Autodesk Inventor part; units mm, degrees
ref_plane "YZ Plane" through (0, 0, 0) normal (1, 0, 0) x (0, 1, 0)
ref_plane "XZ Plane" through (0, 0, 0) normal (0, 1, 0) x (-1, 0, 0)
ref_plane "XY Plane" through (0, 0, 0) normal (0, 0, 1) x (1, 0, 0)
sketch "Esquisse1" plane through (0, 0, 0) normal (0, 0, 1) x (1, 0, 0)
  circle A0 centre (0, 0) radius 63
  circle A1 centre (0, 0) radius 60
  circle A2 centre (0, 0) radius 54
  line L0 (-25.9421, 2.5) -> (-53.9421, 2.5)
  line L1 (-25.9421, -2.5) -> (-53.9421, -2.5)
  line L2 (-20.9421, 0) -> (-20.9421, 14.5)
  line L3 (-25.9421, 14.5) -> (-25.9421, 2.5)
  line L4 (-20.9421, 0) -> (-20.9421, -14.5)
  line L5 (-25.9421, -14.5) -> (-25.9421, 2.5)
  arc A3 (-25.9421, -14.5) -> (-20.9421, -14.5) centre (-23.4421, -14.5) ccw
  arc A4 (-20.9421, 14.5) -> (-25.9421, 14.5) centre (-23.4421, 14.5) ccw
  line L6 (0, 0) -> (0, 11.8583)
  line L7 (25.9421, 2.5) -> (53.9421, 2.5)
  line L8 (25.9421, -2.5) -> (53.9421, -2.5)
  line L9 (20.9421, 0) -> (20.9421, 14.5)
  line L10 (25.9421, 14.5) -> (25.9421, 2.5)
  line L11 (20.9421, 0) -> (20.9421, -14.5)
  line L12 (25.9421, -14.5) -> (25.9421, 14.5)
  arc A5 (20.9421, -14.5) -> (25.9421, -14.5) centre (23.4421, -14.5) ccw
  arc A6 (25.9421, 14.5) -> (20.9421, 14.5) centre (23.4421, 14.5) ccw
  line L13 (25.9421, 2.5) -> (56.5559, 2.5)
  line L14 (56.5559, 2.5) -> (56.5559, -2.5)
  line L15 (56.5559, -2.5) -> (25.9421, -2.5)
  line L16 (25.9421, -2.5) -> (25.9421, 2.5)
  dimension "d0" = 126
  dimension "d1" = 120
  dimension "d2" = 108
  dimension "d3" = 28
  dimension "d6" = 14.5
  dimension "d8" = 5
extrude "Extrusion1" add sketch "Esquisse1" along normal blind 5 contours A0
extrude "Extrusion2" add sketch "Esquisse1" along normal blind 1.7 contours A1 | A2 L8 L12 L7 | A2 L13 L14 L15 | L0 L5 L1 A2
sketch "Esquisse3" plane through (0, 0, 0) normal (0, 0, -1) x (-1, 0, 0)
  line L0 (20.9421, 0) -> (20.9421, 14.5)
  line L1 (20.9421, 0) -> (20.9421, -14.5)
  arc A0 (20.9421, -14.5) -> (25.9421, -14.5) centre (23.4421, -14.5) ccw
  line L2 (25.9421, -14.5) -> (25.9421, 2.5)
  line L3 (25.9421, 14.5) -> (25.9421, 2.5)
  arc A1 (25.9421, 14.5) -> (20.9421, 14.5) centre (23.4421, 14.5) ccw
  arc A2 (-20.9421, 14.5) -> (-25.9421, 14.5) centre (-23.4421, 14.5) ccw
  line L4 (-25.9421, 14.5) -> (-25.9421, 2.5)
  line L5 (-25.9421, -14.5) -> (-25.9421, 14.5)
  arc A3 (-25.9421, -14.5) -> (-20.9421, -14.5) centre (-23.4421, -14.5) ccw
  line L6 (-20.9421, 0) -> (-20.9421, -14.5)
  line L7 (-20.9421, 0) -> (-20.9421, 14.5)
  point P0 (0, 0)
extrude "Extrusion3" add sketch "Esquisse3" against normal blind 3
fillet "Congé1" radius 1 3 edges at (25.9421, 0, 1.7) (25.9421, -2.5, 0.85) (25.9421, 2.5, 0.85)
fillet "Congé2" radius 1 3 edges at (-25.9421, 0, 1.7) (-25.9421, -2.5, 0.85) (-25.9421, 2.5, 0.85)
fillet "Congé3" radius 1 4 edges at (53.9421, 2.5, 0.85) (53.9421, -2.5, 0.85) (-53.9421, 2.5, 0.85) (-53.9421, -2.5, 0.85)
sketch "Esquisse4" plane through (0, 0, 0) normal (0, 0, -1) x (-1, 0, 0)
  arc A0 (53.8821, 3.566) -> (-53.8821, 3.566) centre (0, 0) ccw
  arc A1 (-53.8821, -3.566) -> (53.8821, -3.566) centre (0, 0) ccw
  arc A2 (53.8821, 3.566) -> (-53.8821, 3.566) centre (0, 0) ccw
  arc A3 (52.8843, 2.5) -> (53.8821, 3.566) centre (52.8843, 3.5) ccw
  line L0 (52.8843, 2.5) -> (26.9421, 2.5)
  arc A4 (25.9421, 3.5) -> (26.9421, 2.5) centre (26.9421, 3.5) ccw
  line L1 (25.9421, 3.5) -> (25.9421, 14.5)
  arc A5 (25.9421, 14.5) -> (20.9421, 14.5) centre (23.4421, 14.5) ccw
  line L2 (20.9421, 14.5) -> (20.9421, -14.5)
  arc A6 (20.9421, -14.5) -> (25.9421, -14.5) centre (23.4421, -14.5) ccw
  line L3 (25.9421, -14.5) -> (25.9421, -3.5)
  arc A7 (26.9421, -2.5) -> (25.9421, -3.5) centre (26.9421, -3.5) ccw
  line L4 (26.9421, -2.5) -> (52.8843, -2.5)
  arc A8 (53.8821, -3.566) -> (52.8843, -2.5) centre (52.8843, -3.5) ccw
  arc A9 (-53.8821, -3.566) -> (53.8821, -3.566) centre (0, 0) ccw
  arc A10 (-52.8843, -2.5) -> (-53.8821, -3.566) centre (-52.8843, -3.5) ccw
  line L5 (-26.9421, -2.5) -> (-52.8843, -2.5)
  arc A11 (-25.9421, -3.5) -> (-26.9421, -2.5) centre (-26.9421, -3.5) ccw
  line L6 (-25.9421, -3.5) -> (-25.9421, -14.5)
  arc A12 (-25.9421, -14.5) -> (-20.9421, -14.5) centre (-23.4421, -14.5) ccw
  line L7 (-20.9421, -14.5) -> (-20.9421, 14.5)
  arc A13 (-20.9421, 14.5) -> (-25.9421, 14.5) centre (-23.4421, 14.5) ccw
  line L8 (-25.9421, 14.5) -> (-25.9421, 3.5)
  arc A14 (-26.9421, 2.5) -> (-25.9421, 3.5) centre (-26.9421, 3.5) ccw
  line L9 (-52.8843, 2.5) -> (-26.9421, 2.5)
  arc A15 (-53.8821, 3.566) -> (-52.8843, 2.5) centre (-52.8843, 3.5) ccw
  circle A16 centre (0, 0) radius 63
  line L10 (32.9786, 41.9728) -> (-33, 41.9728)
  line L11 (-33, 41.9728) -> (-33, -42)
  line L12 (-33, -42) -> (32.9786, -42)
  line L13 (32.9786, -42) -> (32.9786, 41.9728)
  line L14 (32.9786, 32.8) -> (-33, 32.8)
  line L15 (32.9786, -32.8) -> (-33, -32.8)
  line L16 (-33.3624, -42.4612) -> (38.9228, 49.5381)
  line L17 (33.3492, -42.4716) -> (-38.936, 49.5277)
  line L18 (-33.2831, 42.3332) -> (-36.4284, 39.8619)
  line L19 (-33.2831, 42.3332) -> (-30.1379, 44.8045)
  arc A17 (-30.1379, 44.8045) -> (-36.4284, 39.8619) centre (-32.5624, 41.4158) ccw
  line L20 (33.2707, 42.3445) -> (30.1254, 44.8158)
  line L21 (33.2707, 42.3445) -> (36.416, 39.8733)
  line L22 (33.2831, -42.3332) -> (36.4284, -39.8619)
  line L23 (33.2831, -42.3332) -> (30.1379, -44.8045)
  arc A18 (30.1379, -44.8045) -> (36.4284, -39.8619) centre (32.5624, -41.4158) ccw
  arc A19 (36.416, 39.8733) -> (30.1254, 44.8158) centre (32.5499, 41.4272) ccw
  line L24 (-33.2707, -42.3445) -> (-36.416, -39.8733)
  arc A20 (-36.416, -39.8733) -> (-30.1254, -44.8158) centre (-32.5499, -41.4272) ccw
  line L25 (-33.2707, -42.3445) -> (-30.1254, -44.8158)
  arc A21 (-53.8821, -3.566) -> (53.8821, -3.566) centre (0, 0) ccw
  line L26 (-38.5851, -37.7782) -> (-27.5766, -46.4277)
  arc A22 (-38.5851, -37.7782) -> (-27.5766, -46.4277) centre (-31.4173, -39.9857) ccw
  line L27 (-38.5969, 37.7661) -> (-27.5885, 46.4156)
  arc A23 (-27.5885, 46.4156) -> (-38.5969, 37.7661) centre (-31.4292, 39.9736) ccw
  line L28 (27.5621, -46.4363) -> (38.5705, -37.7868)
  arc A24 (27.5621, -46.4363) -> (38.5705, -37.7868) centre (31.4028, -39.9943) ccw
  line L29 (27.5766, 46.4277) -> (38.5851, 37.7782)
  arc A25 (38.5851, 37.7782) -> (27.5766, 46.4277) centre (31.4173, 39.9857) ccw
  point P0 (-35.1366, 44.6921)
  point P1 (35.1242, 44.7035)
  point P2 (33, -41.9728)
  point P3 (35.1366, -44.6921)
  point P4 (-32.9786, -41.9728)
  point P5 (-35.1242, -44.7035)
  point P6 (-38.9228, -49.5381)
  dimension "d42" = 33
  dimension "d43" = 42
  dimension "d44" = 4
  dimension "d45" = 4
  dimension "d46" = 3
  dimension "d47" = 65.9786
  dimension "d48" = 83.9728
  dimension "d53" = 4
  dimension "d54" = 4
  dimension "d55" = 3
  dimension "d58" = 360
  dimension "d62" = 360
  dimension "d80" = 7
  dimension "d81" = 14
  dimension "d82" = 7.5
  dimension "d83" = 14
  dimension "d84" = 7
  dimension "d85" = 7.5
  dimension "d86" = 14
  dimension "d87" = 7
  dimension "d88" = 7.5
  dimension "d89" = 14
  dimension "d90" = 7
  dimension "d91" = 7.5
extrude "Extrusion4" cut sketch "Esquisse4" against normal blind 10 contours L25 A1 L16 | L16 A1 L24 | A20 A1
extrude "Extrusion5" cut sketch "Esquisse4" against normal blind 10 contours L18 A0 L17 | A0 A17 L17 picked at (-34.5217, 42.711)
extrude "Extrusion6" cut sketch "Esquisse4" against normal blind 10 contours L19 L17 A0 | A0 L17 A17 picked at (-33.3576, 43.626)
extrude "Extrusion7" cut sketch "Esquisse4" against normal blind 10 contours L21 L16 A0 | A0 L16 A19 picked at (34.5088, 42.7218)
extrude "Extrusion8" cut sketch "Esquisse4" against normal blind 10 contours A18 A1 | A1 L17 L23 L22 | L17 A1 L23
extrude "Extrusion9" cut sketch "Esquisse4" against normal blind 10 contours L16 L20 A0 | A0 A19 L16 picked at (33.3443, 43.6367)
fillet "Congé4" radius 4 6 edges at (36.416, -39.8733, 0.85) (30.1254, -44.8158, 0.85) (36.4284, 39.8619, 0.85) (-36.416, 39.8733, 0.85) (-30.14, -44.806, 0.85) (-36.4284, -39.8619, 0.85)
extrude "Extrusion10" cut sketch "Esquisse4" against normal blind 10 contours A24 A1 A18 | A1 L22 L23 L17 L28 A24 | L17 L23 A1 L28
extrude "Extrusion11" cut sketch "Esquisse4" against normal blind 10 contours L29 L16 L21 A0 | A0 A19 L16 A25 | L29 A0 L20 L16 | L16 A19 A0 A25
extrude "Extrusion12" cut sketch "Esquisse4" against normal blind 10 contours A23 L27 L17 L19 A0 | A0 A17 L17 A23 | L27 A0 L18 L17 | L17 A17 A0 A23
extrude "Extrusion13" cut sketch "Esquisse4" against normal blind 10 contours L26 A1 L25 L16 | L16 L24 A1 L26 | A22 A1 A20
fillet "Congé5" radius 4 8 edges at (38.5851, -37.7782, 0.85) (27.5766, -46.4277, 0.85) (-27.5621, -46.4363, 0.85) (-38.572, -37.7916, 0.85) (27.5927, 46.4181, 0.85) (38.5969, 37.7661, 0.85) (-38.5851, 37.7782, 0.85) (-27.5766, 46.4277, 0.85)
equation "\"d80\" = 0.5 * d81"
equation "\"d90\" = 0.5 * d89"
properties part number "bumper_modified2" material "Plastique ABS"
The model under review builds one solid part; all positions refer to its coordinate system, in mm. A direction names the side the tool comes from. Give positions to 0.01 mm unless a question says otherwise; leave off trailing zeros. Write each loop counter-clockwise with the first axis right and the second up, starting at its lowest first coordinate (ties: lowest second). Pieces come first, ordered by that corner, then holes. Notation, with made-up numbers: (8.25, 86) -> (40.25, 86) arc R8 cw to (40.25, 93) -> close; hole circle Ø3 at (76, 81.25). An arc over 180 degrees is marked (long way). Put each result on its own line as item: value.
(1) We need section A-A, the plane x = 0. Give the boundary of the cut face in (y, z), and give its area (3 significant figures).
Results are:
outline: (-63, 0) -> (-54, 0) -> (-54, 1.7) -> (-60, 1.7) -> (-60, 5) -> (-63, 5) -> close; (54, 0) -> (63, 0) -> (63, 5) -> (60, 5) -> (60, 1.7) -> (54, 1.7) -> close
area: 50.4 mm²
(2) The part is to be moulded in two halves that separate along Y. For faces 4 (the cylindrical face through (-49.785, 20.915, 0.838)), 5 (the flat face through (-23, 0, 0)), say which applies: pulls with the +Y half, pulls with the -Y half, needs draft (parallel to the pull), parting line crosses it, or undercut.
Results are:
face 4: undercut
face 5: needs draft
(3) For pin 1 Ø2.5 at (x, y) = (-24, -4) entering from +Z; pin 2 Ø1.5 at (y, z) = (-4, 2) entering from +X; pin 3 Ø0.5 at (x, z) = (-41, 1) entering from -Y, all flat-tipped, find the tip position at first contact; note any pin that passes through.
Results are:
pin 1: z = 3
pin 2: x = 62.92
pin 3: y = -48.05
(4) We need section B-B, the plane y = 0. Give the boundary of the cut face in (x, z).
Results are:
outline: (-63, 0) -> (-20.94, 0) -> (-20.94, 3) -> (-25.94, 3) -> (-25.94, 2.7) arc R1 cw to (-26.94, 1.7) -> (-60, 1.7) -> (-60, 5) -> (-63, 5) -> close; (20.94, 0) -> (63, 0) -> (63, 5) -> (60, 5) -> (60, 1.7) -> (26.94, 1.7) arc R1 cw to (25.94, 2.7) -> (25.94, 3) -> (20.94, 3) -> close
(5) We need section C-C, the plane x = -32. Give the boundary of the cut face in (y, z).
Results are:
outline: (-54.27, 0) -> (-47.47, 0) -> (-47.47, 1.7) -> (-50.75, 1.7) -> (-50.75, 5) -> (-54.27, 5) -> close; (-2.5, 0) -> (2.5, 0) -> (2.5, 1.7) -> (-2.5, 1.7) -> close; (47.46, 0) -> (54.27, 0) -> (54.27, 5) -> (50.75, 5) -> (50.75, 1.7) -> (47.46, 1.7) -> close
(6) Tool access review of faces 1 (the cylindrical face through (-59.94, -2.64, 3.33)), 2 (the flat face through (56, -23, 5)), 3 (the cylindrical face through (-23.4, -17, 1.5)): name each direction out of +Z, -Z, +X, -X, +Y, -Y from which nothing blocks a thin tool from reaching the whole face with its end or side.
Results are:
face 1: +Z
face 2: +Z, +X, -X, +Y, -Y
face 3: +Z, -Z
(7) To check wall thickness, follow probe 1 along Y at (x, z) = (-22, 1.05); probe 2 along Y at (x, z) = (0, 2.6); probe 3 along X at (y, z) = (-54, 4.55). State the ranges of each line that lie inside material, in increasing order. Write a range as from..to.
Results are:
probe 1: -59.03..-49.32, -16.54..16.54, 49.32..59.03
probe 2: -63..-60, 60..63
probe 3: -32.45..-26.15, 26.15..32.45
(8) We need section D-D, the plane y = -49.5. Give the boundary of the cut face in (x, z).
Results are:
outline: (-38.97, 0) -> (-21.58, 0) -> (-21.58, 1.7) -> (-33.91, 1.7) -> (-33.91, 5) -> (-38.97, 5) -> close; (21.58, 0) -> (38.97, 0) -> (38.97, 5) -> (33.91, 5) -> (33.91, 1.7) -> (21.58, 1.7) -> close
